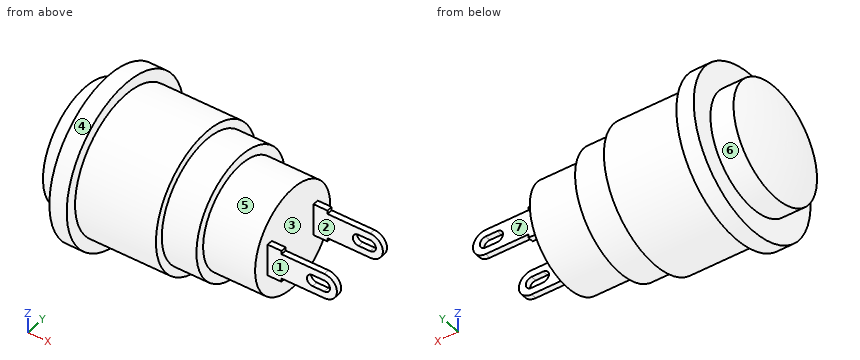
from build123d import *

# Parameters (mm, degrees)
BOSS_EXTRUDE1_DEPTH = 0.5


with BuildPart() as part:
    # Sketch1 → Revolve1 (revolve)
    with BuildSketch(Plane(origin=(0, 0, 0), x_dir=(1, 0, 0), z_dir=(0, 1, 0)), mode=Mode.PRIVATE) as revolve1_sk:
        Polygon((-8, 0), (8, 0), (8, 4.5), (3.5, 4.5), (3.5, 5.3), (0.5, 5.3), (0.5, 6), (-6.5, 6), (-6.5, 7), (-8, 7), align=None)
    revolve(revolve1_sk.sketch.rotate(Axis((-8, 0, 0), (1, 0, 0)), 180), axis=Axis((-8, 0, 0), (1, 0, 0)))

    # Sketch2 → Revolve2 (revolve)
    with BuildSketch(Plane(origin=(0, 0, 0), x_dir=(1, 0, 0), z_dir=(0, 1, 0))):
        with BuildLine():
            Line((-8, 0), (-11, 0))
            add(Edge.make_bspline(
                [(-11, 0), (-11, 2.651487421), (-10, 5)],
                knots=[0, 0, 0, 1, 1, 1], degree=2))
            Line((-10, 5), (-8, 5))
            Line((-8, 5), (-8, 0))
        make_face()
    revolve(axis=Axis((-8, 0, 0), (-1, 0, 0)))

    # Sketch3 → Boss-Extrude1 (add)
    with BuildSketch(Plane(origin=(0, 3, 0), x_dir=(1, 0, 0), z_dir=(0, 1, 0))):
        with BuildLine():
            Line((8, -1.4), (8, 1.4))
            Line((8, 1.4), (9.2, 1.4))
            Line((9.2, 1.4), (9.2, 1.1))
            Line((9.2, 1.1), (12.9, 1.1))
            ThreePointArc((12.9, 1.1), (14, 0), (12.9, -1.1))
            Line((12.9, -1.1), (9.2, -1.1))
            Line((9.2, -1.1), (9.2, -1.4))
            Line((9.2, -1.4), (8, -1.4))
        make_face()
        with BuildLine():
            Line((11.9, 0.5), (12.9, 0.5))
            ThreePointArc((12.9, 0.5), (13.4, 0), (12.9, -0.5))
            Line((12.9, -0.5), (11.9, -0.5))
            ThreePointArc((11.9, -0.5), (11.4, 0), (11.9, 0.5))
        make_face(mode=Mode.SUBTRACT)
    boss_extrude1 = extrude(amount=-BOSS_EXTRUDE1_DEPTH)

    # Mirror1: Boss-Extrude1 across plane
    add(boss_extrude1.mirror(Plane.ZX))


solid = part.part
Verification items for the finished model (mm, model axes). Face numbers are marked on the shaded views. A direction names the side the tool comes from. Coordinates: 2 decimals unless noted, no trailing zeros. Order: outer loops, then holes, each group sorted by start corner. A loop starts at its lowest first (then second) coordinate and runs counter-clockwise, first axis right, second up. Notation, with made-up numbers: M 84.5,88 L 132.5,88 A20 ccw 132.5,101 Z; hole C 82,45.25 d3. An arc over 180 degrees is marked long. One line per item, written item: value. Start each with the question number.
Item 1: Scan lines: probe 1 along X at (y, z) = (4, 5.5); probe 2 along X at (y, z) = (-5, 0.75); probe 3 along Y at (x, z) = (1.5, -4.75). Record each from-to range of solid material in increasing order.
Item 2: Mould release check, pull along Y, two halves, no side actions. Record for the marked faces 1, 2, 3 and 4: released by +Y, released by -Y, zero draft, split by the parting line, or undercut.
Item 3: Sectioned sample at A-A (x = 6). Enter the section's corners in (y, z), then the cut area to 3 significant figures.
Item 4: Gauge pin test, flat ends, axial feed: pin 1 (0.6 mm diameter, centred on x = 8.5, y = -3, fed in from -Z); pin 2 (0.6 mm diameter, centred on x = 12.5, y = 2.5, fed in from +Z); pin 3 (0.8 mm diameter, centred on x = 11.5, z = -0.5, fed in from -Y); pin 4 (7 mm diameter, centred on y = -2, z = -2.5, fed in from +X). Record the tip position at first contact, or that the pin passes through.
Item 5: Access from +Z, -Z, +X, -X, +Y, -Y to the whole of each face (thin tool, end or side, straight path). Record for the marked faces 5, 6 and 7.
Conclusion:
1. probe 1: x = -8 to -6.5
1. probe 2: x = -8 to 3.5
1. probe 3: y = -2.35 to 2.35
2. face 1: released by -Y
2. face 2: undercut
2. face 3: undercut
2. face 4: split by the parting line
3. outline: C 0,0 d9
3. area: 63.6 mm^2
4. pin 1: stops at z = -1.4
4. pin 2: stops at z = 1.1
4. pin 3: stops at y = -3
4. pin 4: stops at x = 14
5. face 5: +X
5. face 6: -X
5. face 7: +Z, -Z, +X, +Y
